Build history of the part. All positions in model axes, mm. A direction names the side the tool comes from. Give positions to 0.01 mm unless a question says otherwise; leave off trailing zeros. Order: outer loops, then holes, each group sorted by start corner. A loop starts at its lowest first (then second) coordinate and runs counter-clockwise, first axis right, second up. Notation, with made-up numbers: (80.5, -4.75) -> (121.5, -4.75) arc R22 ccw to (121.5, 6.25) -> close; hole circle Ø6 at (12.5, 60). An arc over 180 degrees is marked (long way). Use a Markdown table: item, result. Add a question column.
```python
from build123d import *

# Parameters (mm, degrees)
F0_W     = 790.575
F0_H     = 496.8875
F1_DEPTH = 76.2
F2_SIZE2 = 4.7625
F2_SIZE  = 26.9875
F4_START = -248.44475
F4_DEPTH = 496.8895


with BuildPart() as f1:
    # F0 (on Front) → F1 (new body)
    with BuildSketch(Plane.XZ):
        Rectangle(F0_W, F0_H)
        with BuildLine():
            Line((-298.45, -57.94375), (298.45, -57.94375))
            ThreePointArc((298.45, -57.94375), (302.9401280605, -59.8036219395), (304.8, -64.29375))
            Line((304.8, -64.29375), (304.8, -165.89375))
            ThreePointArc((304.8, -165.89375), (302.9401280605, -170.3838780605), (298.45, -172.24375))
            Line((298.45, -172.24375), (-298.45, -172.24375))
            ThreePointArc((-298.45, -172.24375), (-302.9401280605, -170.3838780605), (-304.8, -165.89375))
            Line((-304.8, -165.89375), (-304.8, -64.29375))
            ThreePointArc((-304.8, -64.29375), (-302.9401280605, -59.8036219395), (-298.45, -57.94375))
        make_face(mode=Mode.SUBTRACT)
        with BuildLine():
            Line((-298.45, 167.48125), (298.45, 167.48125))
            ThreePointArc((298.45, 167.48125), (302.9401280605, 165.6213780605), (304.8, 161.13125))
            Line((304.8, 161.13125), (304.8, 21.43125))
            ThreePointArc((304.8, 21.43125), (302.9401280605, 16.9411219395), (298.45, 15.08125))
            Line((298.45, 15.08125), (-298.45, 15.08125))
            ThreePointArc((-298.45, 15.08125), (-302.9401280605, 16.9411219395), (-304.8, 21.43125))
            Line((-304.8, 21.43125), (-304.8, 161.13125))
            ThreePointArc((-304.8, 161.13125), (-302.9401280605, 165.6213780605), (-298.45, 167.48125))
        make_face(mode=Mode.SUBTRACT)
    extrude(amount=-F1_DEPTH)

    # F2
    f2_edges = [f1.edges().sort_by_distance(p)[0] for p in [
        (-395.2875, 0, 0),
        (395.2875, 0, 0),
    ]]
    f2_side = f1.faces().sort_by_distance((0, 0, -2.004685))[0]
    chamfer(f2_edges, length=F2_SIZE, length2=F2_SIZE2, reference=f2_side)

    # F3 (on Top) → F4 (intersect)
    with BuildSketch(Plane.XY.offset(F4_START)):
        Polygon((-395.2875, 4.7625), (-368.3, 0), (368.3, 0), (395.2875, 4.7625), (395.0116157824, 6.3258438996), (368.1610003512, 1.5875), (-368.1610003512, 1.5875), (-395.0116157824, 6.3258438996), align=None)
    extrude(amount=F4_DEPTH, mode=Mode.INTERSECT)


solid = f1.part
```
(1) Tool access for faces 5 (the face through (381.983, 2.415, -3.478)), 6 (the face through (5, 1.588, -3)): list every direction of +Z, -Z, +X, -X, +Y, -Y with a clear straight run to the whole face (end or side of a thin tool).
(2) Band-saw the part on C-C on z = -194.5. Give the cut face in (x, y), plus the area to 3 significant figures.
(3) Mould opens along X. For faces 1 (the face through (-381.983, 2.415, -3.478)), 2 (the face through (381.77, 3.99, -3.48)), 3 (the face through (-381.398, 3.924, -3.478)), 4 (the face through (-5, 0, 3)) say: released by +X, released by -X, zero draft, split by the parting line, or undercut.
(4) Pin check, flat tips, straight feed: pin 1 Ø8 at (x, z) = (243.5, 172) entering from +Y; pin 2 Ø3 at (x, y) = (-263.5, 3.5) entering from -Z. Stop position of each tip, or through.
(5) Band-saw the part on B-B on x = -199.5. Give the cut face in (y, z), plus the area to 3 significant figures.
(6) Wall check: probe 1 along Z at (x, y) = (169, 0.75); probe 2 along Y at (x, z) = (355, -179). Give the ranges that are in metal, low to high.
(7) Band-saw the part on D-D on y = 2.75. Give the cut face in (x, z), plus the area to 3 significant figures.
(8) Band-saw the part on A-A on z = 69. Give the cut face in (x, y), plus the area to 3 significant figures.
Response:
| question | item | result |
|---|---|---|
| 1 | face 5 | +Z, -Z, +X, -Y |
| 1 | face 6 | +Z, -Z, +Y |
| 2 | outline | (-395.29, 4.76) -> (-368.3, 0) -> (368.3, 0) -> (395.29, 4.76) -> (395.01, 6.33) -> (368.16, 1.59) -> (-368.16, 1.59) -> (-395.01, 6.33) -> close |
| 2 | area | 1,260 mm² |
| 3 | face 1 | released by -X |
| 3 | face 2 | undercut |
| 3 | face 3 | undercut |
| 3 | face 4 | zero draft |
| 4 | pin 1 | stops at y = 1.59 |
| 4 | pin 2 | passes through |
| 5 | outline | (0, -248.44) -> (1.59, -248.44) -> (1.59, -172.24) -> (0, -172.24) -> close; (0, -57.94) -> (1.59, -57.94) -> (1.59, 15.08) -> (0, 15.08) -> close; (0, 167.48) -> (1.59, 167.48) -> (1.59, 248.44) -> (0, 248.44) -> close |
| 5 | area | 365 mm² |
| 6 | probe 1 | z = -248.44 to -172.24, -57.94 to 15.08, 167.48 to 248.44 |
| 6 | probe 2 | y = 0 to 1.59 |
| 7 | outline | (-383.88, -248.44) -> (-374.75, -248.44) -> (-374.75, 248.44) -> (-383.88, 248.44) -> close; (374.75, -248.44) -> (383.88, -248.44) -> (383.88, 248.44) -> (374.75, 248.44) -> close |
| 7 | area | 9,080 mm² |
| 8 | outline | (-395.29, 4.76) -> (-368.3, 0) -> (-304.8, 0) -> (-304.8, 1.59) -> (-368.16, 1.59) -> (-395.01, 6.33) -> close; (304.8, 0) -> (368.3, 0) -> (395.29, 4.76) -> (395.01, 6.33) -> (368.16, 1.59) -> (304.8, 1.59) -> close |
| 8 | area | 288 mm² |
